Answer from the drawing. Dimensions are ordinates in mm from the lowest x, y and z of the part. Coordinates: 2 decimals unless noted, no trailing zeros. Loops run counter-clockwise (first coordinate to the right, second up) from the corner with the lowest first, then second, coordinate; pieces in that order, holes last.
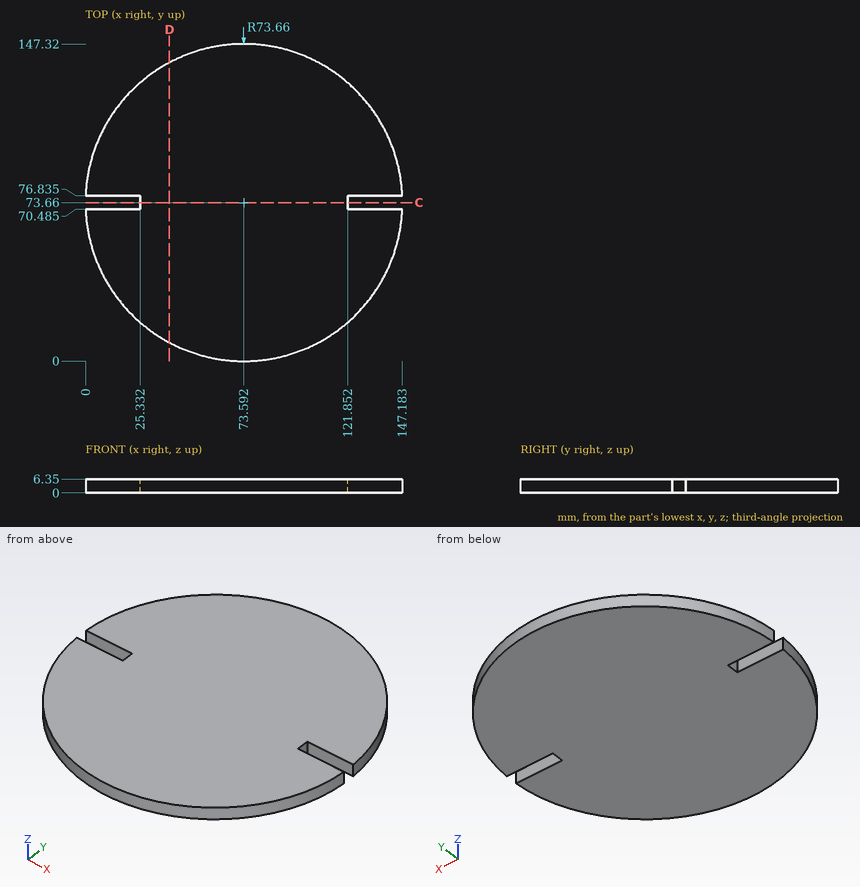
Item 1: A cutting plane is placed at C-C on y = 73.66. Determine the outline of the cut face in (x, z).
Numbers:
outline: (25.33, 0) - (121.85, 0) - (121.85, 6.35) - (25.33, 6.35) - close
Item 2: A cutting plane is placed at D-D on x = 39. Determine the outline of the cut face in (y, z).
Numbers:
outline: (8.63, 0) - (138.69, 0) - (138.69, 6.35) - (8.63, 6.35) - close
Item 3: Given pin 1 (8 mm diameter, centred on x = 38, y = 79, fed in from -Z); pin 2 (3 mm diameter, centred on x = 24, z = 3.5, fed in from -Y) (1 decimal); pin 3 (1 mm diameter, centred on y = 94.5, z = 5.5, fed in from +X); pin 4 (1.9 mm diameter, centred on x = 15, z = 2, fed in from +Y), each flat-ended and moving along its own axis, determine where each tip first touches the part or whether it passes through.
Numbers:
pin 1: stops at z = 0
pin 2: stops at y = 17.9
pin 3: stops at x = 144.39
pin 4: stops at y = 119.52
Item 4: Find the intervals of material crossed by line 1 along Y through (x, z) = (22, 0.5) (1 decimal); line 2 along X through (y, z) = (41.5, 3.5); line 3 along X through (y, z) = (28.5, 4.5) (1 decimal), in increasing order.
Numbers:
line 1: y = 21.1 to 70.5, 76.8 to 126.2
line 2: x = 7.32 to 139.86
line 3: x = 15.4 to 131.8
